Here's how the part is built. I have some questions about the finished solid (model axes, mm). A direction names the side the tool comes from. Give positions to 0.01 mm unless a question says otherwise; leave off trailing zeros. Write each loop counter-clockwise with the first axis right and the second up, starting at its lowest first coordinate (ties: lowest second). Pieces come first, ordered by that corner, then holes. Notation, with made-up numbers: (-27.5, -39.75) -> (20.5, -39.75) arc R20 cw to (20.5, -11.75) -> close; hole circle Ø1 at (-31, 89). An arc over 180 degrees is marked (long way). Return JSON: item names as keys, results as strings.
from build123d import *

# Parameters (mm, degrees)
F1_DEPTH       = 82.55
F2_F1_R        = 5.08
F2_F2_R        = 5.08
F4_D           = 4.826
F4_DEPTH       = 25.4
F4_TIP         = 1.4498766737
F6_D           = 6.35
F6_DEPTH       = 25.4
F6_TIP         = 1.9077324654
F8_D           = 6.35
F8_DEPTH       = 25.4
F8_START       = 0.3707141
F8_CBORE_D     = 12.7
F8_CBORE_DEPTH = 6.35
F8_TIP         = 1.9077324654


with BuildPart() as f1:
    # F0 (on Front) → F1 (new body)
    with BuildSketch(Plane.XZ):
        Polygon((0, 95.25), (0, 0), (88.2142, 0), (88.2142, 12.7), (44.45, 12.7), (44.45, 95.25), align=None)
    extrude(amount=F1_DEPTH)

    # F2: fillet of radius 5.08 on 8 edges, made by hand

    # F2_f1
    f2_f1_edges = [f1.edges().sort_by_distance(p)[0] for p in [
        (44.45, -41.275, 12.7),
    ]]
    fillet(f2_f1_edges, radius=F2_F1_R)

    # F2_f2
    f2_f2_edges = [f1.edges().sort_by_distance(p)[0] for p in [
        (44.45, -41.275, 95.25),
        (0, -41.275, 95.25),
        (44.45, -82.55, 56.515),
        (44.45, 0, 56.515),
        (0, -82.55, 47.625),
        (0, 0, 47.625),
        (88.2142, -41.275, 12.7),
        (45.9378975516, 0, 14.1878975516),
        (45.9378975516, -82.55, 14.1878975516),
    ]]
    fillet(f2_f2_edges, radius=F2_F2_R)

    # F4
    with Locations(Plane.XY.offset(95.25)):
        with Locations((22.225, -7.9375), (22.225, -74.6125)):
            Hole(F4_D / 2, depth=F4_DEPTH)
            with Locations((0, 0, -(F4_DEPTH + F4_TIP / 2))):  # 118° drill point
                Cone(0, F4_D / 2, F4_TIP, mode=Mode.SUBTRACT)

    # F6
    with Locations(Plane(origin=(0, 0, 0), x_dir=(1, 0, 0), z_dir=(0, 0, -1))):
        with Locations((12.7, 73.025), (12.7, 9.525)):
            Hole(F6_D / 2, depth=F6_DEPTH)
            with Locations((0, 0, -(F6_DEPTH + F6_TIP / 2))):  # 118° drill point
                Cone(0, F6_D / 2, F6_TIP, mode=Mode.SUBTRACT)

    # F8
    # its depths count from where the whole tool has entered the part; down to there all is cleared
    with Locations(Plane.XY.offset(12.7).offset(-F8_START)):
        with Locations((75.5142, -9.525), (75.5142, -73.025)):
            CounterBoreHole(F8_D / 2, F8_CBORE_D / 2, F8_CBORE_DEPTH, depth=F8_DEPTH)
            with Locations((0, 0, -(F8_DEPTH + F8_TIP / 2))):  # 118° drill point
                Cone(0, F8_D / 2, F8_TIP, mode=Mode.SUBTRACT)


solid = f1.part
1. For pin 1 Ø14.5 at (x, y) = (75.51, -9.52) entering from +Z; pin 2 Ø7.5 at (x, y) = (75.51, -73.03) entering from +Z; pin 3 Ø4 at (x, y) = (75.51, -9.52) entering from -Z, each with a flat end and sliding along its axis, tell me the tip position at first contact or that it passes through.
Taken from the geometry:
{"pin 1": "stops at z = 12.7", "pin 2": "stops at z = 5.98", "pin 3": "passes through"}
2. Suppose I cut it at A-A, the plane y = -23.5. List the corners of the cut face in (x, z) for me, and give its area (3 significant figures).
Taken from the geometry:
{"outline": "(0, 0) -> (88.21, 0) -> (88.21, 7.62) arc R5.08 ccw to (83.13, 12.7) -> (49.53, 12.7) arc R5.08 cw to (44.45, 17.78) -> (44.45, 90.17) arc R5.08 ccw to (39.37, 95.25) -> (5.08, 95.25) arc R5.08 ccw to (0, 90.17) -> close", "area": "4,780 mm²"}
3. Suppose I cut it at B-B, the plane z = 48. List the corners of the cut face in (x, y) for me, and give its area (3 significant figures).
Taken from the geometry:
{"outline": "(0, -77.47) arc R5.08 ccw to (5.08, -82.55) -> (39.37, -82.55) arc R5.08 ccw to (44.45, -77.47) -> (44.45, -5.08) arc R5.08 ccw to (39.37, 0) -> (5.08, 0) arc R5.08 ccw to (0, -5.08) -> close", "area": "3,650 mm²"}
4. Suppose I cut it at C-C, the plane x = 57. List the corners of the cut face in (y, z) for me.
Taken from the geometry:
{"outline": "(-82.55, 0) -> (0, 0) -> (0, 7.62) arc R5.08 ccw to (-5.08, 12.7) -> (-77.47, 12.7) arc R5.08 ccw to (-82.55, 7.62) -> close"}
5. If we mould it in two halves opening along X, with no side actions, what happens to faces 1 (the face through (88.214, -41, 4)), 2 (the face through (1.528, -41.853, 93.801)), 3 (the face through (77, -70, 5.979))? For each: released by +X, released by -X, zero draft, split by the parting line, or undercut.
Taken from the geometry:
{"face 1": "released by +X", "face 2": "released by -X", "face 3": "undercut"}
6. Suppose I cut it at D-D, the plane z = 77.5. Count the separate pieces of the cut face and the enclosed holes in it, and give its area (3 significant figures).
Taken from the geometry:
{"separate pieces": "1", "enclosed holes": "2", "area": "3,610 mm²"}
7. Which directions (+Z, -Z, +X, -X, +Y, -Y) give clear straight access to the entire face, cutting with the end or side of a thin tool? Please do faces 4 (the face through (78.686, -9.385, 2.948)), 5 (the face through (78.93, -67.67, 9.39)), 6 (the face through (42.922, -81.101, 57.057)).
Taken from the geometry:
{"face 4": "+Z, -Z", "face 5": "+Z", "face 6": "+Z, +X, -Y"}
8. If I drill on line 1 (Y direction, x = 12.7, z = 5.75); line 2 (Y direction, x = 10.5, z = 25); line 3 (X direction, y = -29, z = 78.5), over which ranges is the centre line in solid material (lowest first)? Write a range as [from, to].
Taken from the geometry:
{"line 1": "y = [-82.55, -76.2], [-69.85, -12.7], [-6.35, 0]", "line 2": "y = [-82.55, -75.31], [-70.74, -11.81], [-7.24, 0]", "line 3": "x = [0, 44.45]"}
